from build123d import *

# Parameters (mm, degrees)
BOSS_EXTRUDE1_DEPTH = 65
FILLET1_R           = 1
CUT_EXTRUDE1_DEPTH  = 66
FILLET2_R           = 0.5
FILLET3_R           = 0.25


with BuildPart() as part:
    # Sketch3 → Boss-Extrude1 (new body)
    with BuildSketch(Plane(origin=(0, 0, 0), x_dir=(1, 0, 0), z_dir=(0, 1, 0))):
        with BuildLine():
            Line((7, 18.5), (7, 19.5))
            ThreePointArc((7, 19.5), (6.646446609, 19.646446609), (6.5, 20))
            Line((6.5, 20), (0, 20))
            Line((0, 20), (0, 13.5))
            ThreePointArc((0, 13.5), (0.353553391, 13.353553391), (0.5, 13))
            Line((0.5, 13), (1.5, 13))
            Line((1.5, 13), (1.5, 16))
            Line((1.5, 16), (3, 16))
            Line((3, 16), (5.5, 13.5))
            Line((5.5, 13.5), (5.5, 10.5))
            Line((5.5, 10.5), (6, 10))
            Line((6, 10), (5.5, 9.5))
            Line((5.5, 9.5), (5.5, 6.5))
            Line((5.5, 6.5), (3, 4))
            Line((3, 4), (1.5, 4))
            Line((1.5, 4), (1.5, 7))
            Line((1.5, 7), (0.5, 7))
            ThreePointArc((0.5, 7), (0.353553391, 6.646446609), (0, 6.5))
            Line((0, 6.5), (0, 0))
            Line((0, 0), (6.5, 0))
            ThreePointArc((6.5, 0), (6.646446609, 0.353553391), (7, 0.5))
            Line((7, 0.5), (7, 1.5))
            Line((7, 1.5), (4, 1.5))
            Line((4, 1.5), (4, 3))
            Line((4, 3), (6.5, 5.5))
            Line((6.5, 5.5), (9.5, 5.5))
            Line((9.5, 5.5), (10, 6))
            Line((10, 6), (10.5, 5.5))
            Line((10.5, 5.5), (13.5, 5.5))
            Line((13.5, 5.5), (16, 3))
            Line((16, 3), (16, 1.5))
            Line((16, 1.5), (13, 1.5))
            Line((13, 1.5), (13, 0.5))
            ThreePointArc((13, 0.5), (13.353553391, 0.353553391), (13.5, 0))
            Line((13.5, 0), (20, 0))
            Line((20, 0), (20, 6.5))
            ThreePointArc((20, 6.5), (19.646446609, 6.646446609), (19.5, 7))
            Line((19.5, 7), (18.5, 7))
            Line((18.5, 7), (18.5, 4))
            Line((18.5, 4), (17, 4))
            Line((17, 4), (14.5, 6.5))
            Line((14.5, 6.5), (14.5, 9.5))
            Line((14.5, 9.5), (14, 10))
            Line((14, 10), (14.5, 10.5))
            Line((14.5, 10.5), (14.5, 13.5))
            Line((14.5, 13.5), (17, 16))
            Line((17, 16), (18.5, 16))
            Line((18.5, 16), (18.5, 13))
            Line((18.5, 13), (19.5, 13))
            ThreePointArc((19.5, 13), (19.646446609, 13.353553391), (20, 13.5))
            Line((20, 13.5), (20, 20))
            Line((20, 20), (13.5, 20))
            ThreePointArc((13.5, 20), (13.353553391, 19.646446609), (13, 19.5))
            Line((13, 19.5), (13, 18.5))
            Line((13, 18.5), (16, 18.5))
            Line((16, 18.5), (16, 17))
            Line((16, 17), (13.5, 14.5))
            Line((13.5, 14.5), (10.5, 14.5))
            Line((10.5, 14.5), (10, 14))
            Line((10, 14), (9.5, 14.5))
            Line((9.5, 14.5), (6.5, 14.5))
            Line((6.5, 14.5), (4, 17))
            Line((4, 17), (4, 18.5))
            Line((4, 18.5), (7, 18.5))
        make_face()
    extrude(amount=BOSS_EXTRUDE1_DEPTH)

    # Fillet1
    fillet1_edges = [part.edges().sort_by_distance(p)[0] for p in [
        (20, 32.5, 0),
        (0, 32.5, 0),
        (0, 32.5, -20),
        (20, 32.5, -20),
    ]]
    fillet(fillet1_edges, radius=FILLET1_R)

    # Sketch4 → Cut-Extrude1 (cut, through all)
    with BuildSketch(Plane(origin=(0, 65, 0), x_dir=(1, 0, 0), z_dir=(0, 1, 0))):
        with BuildLine():
            Line((10, 11), (11.195582496, 12.195582496))
            ThreePointArc((11.195582496, 12.195582496), (10, 12.5), (8.804417504, 12.195582496))
            Line((8.804417504, 12.195582496), (10, 11))
        make_face()
        with BuildLine():
            ThreePointArc((12.195582496, 11.195582496), (11.767766953, 11.767766953), (11.195582496, 12.195582496))
            Line((11.195582496, 12.195582496), (10, 11))
            Line((10, 11), (11, 10))
            Line((11, 10), (12.195582496, 11.195582496))
        make_face()
        with BuildLine():
            Line((9, 10), (10, 11))
            Line((10, 11), (8.804417504, 12.195582496))
            ThreePointArc((8.804417504, 12.195582496), (8.232233047, 11.767766953), (7.804417504, 11.195582496))
            Line((7.804417504, 11.195582496), (9, 10))
        make_face()
        Polygon((11, 10), (10, 11), (9, 10), (10, 9), align=None)
        with BuildLine():
            Line((7.804417504, 8.804417504), (9, 10))
            Line((9, 10), (7.804417504, 11.195582496))
            ThreePointArc((7.804417504, 11.195582496), (7.5, 10), (7.804417504, 8.804417504))
        make_face()
        with BuildLine():
            Line((10, 9), (9, 10))
            Line((9, 10), (7.804417504, 8.804417504))
            ThreePointArc((7.804417504, 8.804417504), (8.232233047, 8.232233047), (8.804417504, 7.804417504))
            Line((8.804417504, 7.804417504), (10, 9))
        make_face()
        with BuildLine():
            Line((11.195582496, 7.804417504), (10, 9))
            Line((10, 9), (8.804417504, 7.804417504))
            ThreePointArc((8.804417504, 7.804417504), (10, 7.5), (11.195582496, 7.804417504))
        make_face()
        with BuildLine():
            Line((12.195582496, 8.804417504), (11, 10))
            Line((11, 10), (10, 9))
            Line((10, 9), (11.195582496, 7.804417504))
            ThreePointArc((11.195582496, 7.804417504), (11.767766953, 8.232233047), (12.195582496, 8.804417504))
        make_face()
        with BuildLine():
            ThreePointArc((12.5, 10), (12.422700584, 10.616864556), (12.195582496, 11.195582496))
            Line((12.195582496, 11.195582496), (11, 10))
            Line((11, 10), (12.195582496, 8.804417504))
            ThreePointArc((12.195582496, 8.804417504), (12.422700584, 9.383135444), (12.5, 10))
        make_face()
        with BuildLine():
            ThreePointArc((8.804417504, 7.804417504), (8.232233047, 8.232233047), (7.804417504, 8.804417504))
            Line((7.804417504, 8.804417504), (7, 8))
            Line((7, 8), (8, 7))
            Line((8, 7), (8.804417504, 7.804417504))
        make_face()
        with BuildLine():
            Line((13, 8), (12.195582496, 8.804417504))
            ThreePointArc((12.195582496, 8.804417504), (11.767766953, 8.232233047), (11.195582496, 7.804417504))
            Line((11.195582496, 7.804417504), (12, 7))
            Line((12, 7), (13, 8))
        make_face()
        with BuildLine():
            Line((13, 12), (12, 13))
            Line((12, 13), (11.195582496, 12.195582496))
            ThreePointArc((11.195582496, 12.195582496), (11.767766953, 11.767766953), (12.195582496, 11.195582496))
            Line((12.195582496, 11.195582496), (13, 12))
        make_face()
        with BuildLine():
            ThreePointArc((7.804417504, 11.195582496), (8.232233047, 11.767766953), (8.804417504, 12.195582496))
            Line((8.804417504, 12.195582496), (8, 13))
            Line((8, 13), (7, 12))
            Line((7, 12), (7.804417504, 11.195582496))
        make_face()
    extrude(amount=-CUT_EXTRUDE1_DEPTH, mode=Mode.SUBTRACT)

    # Fillet2
    fillet2_edges = [part.edges().sort_by_distance(p)[0] for p in [
        (18.5, 32.5, -13),
        (18.5, 32.5, -16),
        (14.5, 32.5, -10.5),
        (14.5, 32.5, -9.5),
        (18.5, 32.5, -4),
        (18.5, 32.5, -7),
        (13, 32.5, -1.5),
        (16, 32.5, -1.5),
        (10.5, 32.5, -5.5),
        (9.5, 32.5, -5.5),
        (4, 32.5, -1.5),
        (7, 32.5, -1.5),
        (1.5, 32.5, -7),
        (1.5, 32.5, -4),
        (5.5, 32.5, -9.5),
        (5.5, 32.5, -10.5),
        (1.5, 32.5, -16),
        (1.5, 32.5, -13),
        (7, 32.5, -18.5),
        (4, 32.5, -18.5),
        (9.5, 32.5, -14.5),
        (10.5, 32.5, -14.5),
        (16, 32.5, -18.5),
        (13, 32.5, -18.5),
    ]]
    fillet(fillet2_edges, radius=FILLET2_R)

    # Fillet3
    fillet3_edges = [part.edges().sort_by_distance(p)[0] for p in [
        (7, 32.5, -12),
        (8, 32.5, -13),
        (12, 32.5, -13),
        (13, 32.5, -12),
        (13, 32.5, -8),
        (12, 32.5, -7),
        (8, 32.5, -7),
        (7, 32.5, -8),
    ]]
    fillet(fillet3_edges, radius=FILLET3_R)


solid = part.part
CAD build for the part. Positions are in the model's coordinates, mm. A direction names the side the tool comes from. Round coordinates to 2 decimals unless told otherwise and drop trailing zeros. Put each result on its own line as item: value. Start each with the question number.
1) 3-axis set-ups, long thin cutter, end or side, ignore diameter. For faces 4 (the flat face through (14, 65, -8)), 5 (the flat face through (16, 32, -15)): which of +Z, -Z, +X, -X, +Y, -Y reach the whole face in a straight line?
2) Drill centre lines: probe 1 along X at (y, z) = (36, -17.25); probe 2 along Z at (x, y) = (4.5, 37); probe 3 along Z at (x, y) = (17, 25). Where is each one in solid material? Low to high. Write a range as [from, to].
3) Pull direction X, two halves, no side cores. Call faces 1 (the flat face through (15, 32, -4)), 2 (the flat face through (16, 32, -20)), 3 (the flat face through (0, 32, -4)): pulls with the +X half, pulls with the -X half, needs draft (parallel to the pull), parting line crosses it, or undercut.
4) Pin check, flat tips, straight feed: pin 1 Ø0.8 at (y, z) = (21, -12.5) entering from +X; pin 2 Ø3 at (y, z) = (23.5, -12.5) entering from +X; pin 3 Ø0.8 at (x, y) = (12, 37.5) entering from -Z; pin 4 Ø1.4 at (y, z) = (33.5, -12.5) entering from -X. Stop position of each tip, or through.
Resolved:
1. face 4: +Z, -Z, +X, -X, +Y
1. face 5: +Y, -Y
2. probe 1: [0, 4], [16, 20]
2. probe 2: [-20, -18.5], [-16.5, -14.5], [-5.5, -3.5], [-1.5, 0]
2. probe 3: [-20, -16], [-4, 0]
3. face 1: undercut
3. face 2: needs draft
3. face 3: pulls with the -X half
4. pin 1: x = 14.5
4. pin 2: x = 20
4. pin 3: z = -14.5
4. pin 4: x = 0.46
